Autodesk Inventor part; units mm, degrees
ref_plane "YZ Plane" through (0, 0, 0) normal (1, 0, 0) x (0, 1, 0)
ref_plane "XZ Plane" through (0, 0, 0) normal (0, 1, 0) x (-1, 0, 0)
ref_plane "XY Plane" through (0, 0, 0) normal (0, 0, 1) x (1, 0, 0)
sketch "Skizze1" plane through (0, 0, 0) normal (0, 1, 0) x (-1, 0, 0)
  line L0 (0, 0) -> (0, 3)
  line L1 (0, 3) -> (-8, 3)
  line L2 (-8, 3) -> (-8, 4.5)
  line L3 (-10.5, 7) -> (-22.5, 7)
  line L4 (-22.5, 7) -> (-22.5, 0)
  line L5 (-22.5, 0) -> (0, 0)
  arc A0 (-8, 4.5) -> (-10.5, 7) centre (-10.5, 4.5) ccw
  point P0 (-8, 7)
  dimension "d0" = 6
  dimension "d1" = 8
  dimension "d2" = 14.5
  dimension "d3" = 14
  dimension "d4" = 2.5
revolve "Umdrehung1" add sketch "Skizze1" angle 360 about axis through (22.5, 0, 0) along (-1, 0, 0)
thread "Gewinde1"
sketch "Skizze2" plane through (0, 0, 0) normal (0, 1, 0) x (-1, 0, 0)
  line L0 (0, 0) -> (-22.5, 0)
  line L1 (-22.5, -7) -> (-22.5, 7)
  line L2 (0, -1.5) -> (-9.5, -1.5)
  line L3 (0, -1.5) -> (0, 0)
  line L4 (0, -3) -> (0, 3)
  line L5 (-11, -5) -> (-22.5, -5)
  line L6 (-9.5, -1.5) -> (-11, -5)
  line L7 (-22.5, -5) -> (-22.5, 0)
  dimension "d8" = 3
  dimension "d9" = 9.5
  dimension "d12" = 10
  dimension "d13" = 11.5
revolve "Umdrehung2" cut sketch "Skizze2" angle 360 about axis through (0, 0, 0) along (1, 0, 0)
fillet "Rundung1" radius 2 1 edges at (11, 0, 5)
thread "Gewinde2"
properties part number "1071"
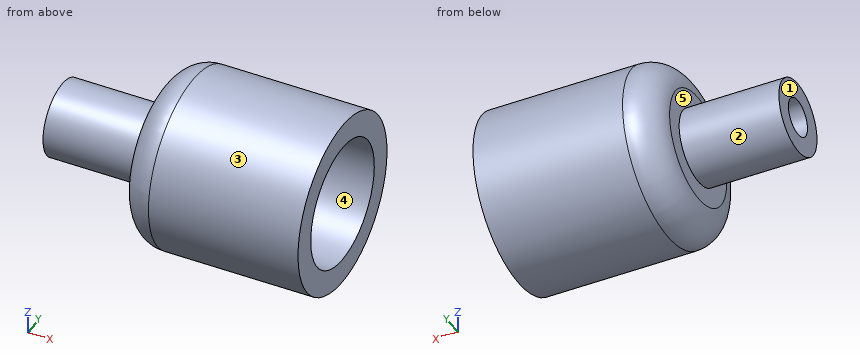
Source: CAD feature listing. Evaluate the final solid. Frame: model axes, mm. Face numbers are marked on the shaded views. A direction names the side the tool comes from. Coordinates: 2 decimals unless noted, no trailing zeros. Write each loop counter-clockwise with the first axis right and the second up, starting at its lowest first coordinate (ties: lowest second). Pieces come first, ordered by that corner, then holes. Notation, with made-up numbers: (11, 5) -> (43, 5) arc R30 ccw to (43, 36) -> close; hole circle Ø8 at (12, -7.75). An arc over 180 degrees is marked (long way). Return JSON: item names as keys, results as strings. Group by question number.
1) Section query A-A, the plane x = 17.25. Return loops of the section in (y, z), plus the area to 3 significant figures.
2) Section query B-B, the plane x = 3. Return loops of the section in (y, z), plus the area to 3 significant figures.
3) Ray query, line 1 along Y through (x, z) = (20.25, 0); line 2 along Y through (x, z) = (4.25, 0); line 3 along X through (y, z) = (-0.5, -3.75). Return the intervals inside material, ascending.
4) Mould query, pull axis Z, two halves, no side actions, for the marked faces 3, 4 and 5. Classes: +Z half, -Z half, draft (parallel to the pull), parting line (faces both ways), or undercut.
5) Contact query for flat-ended pins moving along their axis: P1, Ø8, axis at x = 13.5, z = 4, coming from the +Y side; P2, Ø4, axis at x = 2.5, z = -4, coming from the -Y side; P3, Ø4, axis at x = 13, z = 5, coming from the +Y side; P4, Ø5, axis at x = 10, z = -5, coming from the -Y side. Output: stop coordinate, or through.
6) Set-up query: the marked faces 1 and 2. Return all of +Z, -Z, +X, -X, +Y, -Y with unobstructed straight access to the full face (end or side cutting, diameter ignored); none if empty.
From the geometry:
{
 "1": {"outline": "circle Ø14 at (0, 0); hole circle Ø10 at (0, 0)", "area": "75.4 mm²"},
 "2": {"outline": "circle Ø6 at (0, 0); hole circle Ø3 at (0, 0)", "area": "21.2 mm²"},
 "3": {"line 1": "-7 to -5, 5 to 7", "line 2": "-3 to -1.5, 1.5 to 3", "line 3": "8 to 10.48"},
 "4": {"face 3": "parting line", "face 4": "undercut", "face 5": "draft"},
 "5": {"P1": "y = 7", "P2": "y = -2.24", "P3": "y = 6.32", "P4": "y = -6.52"},
 "6": {"face 1": "+Z, -Z, -X, +Y, -Y", "face 2": "-X"}
}
